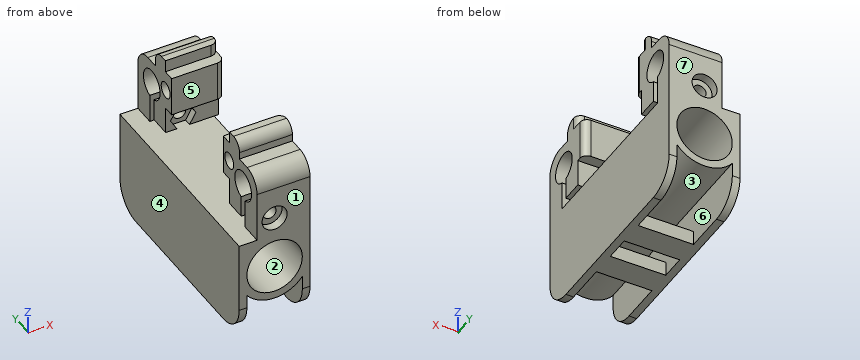
```python
from build123d import *

# Parameters (mm, degrees)
SKETCH_1_W                = 15.5
SKETCH_1_H                = 11.302783866
EXTRUDE_1_DEPTH           = 60
SKETCH_2_R                = 4.2
CUT_EXTRUDE_1_DEPTH       = 90
CUT_EXTRUDE_2_DEPTH       = 40
SKETCH_4_W                = 15.5
SKETCH_4_H                = 19.5
SKETCH_4_H_2              = 7
CUT_EXTRUDE_3_DEPTH       = 6
FILLET_1_R                = 5
FILLET_2_R                = 8
SKETCH_13_R               = 1.8
CUT_EXTRUDE_9_DEPTH       = 75
CUT_EXTRUDE_10_DEPTH      = 34
CUT_EXTRUDE_10_DEPTH_BACK = 2
SKETCH_15_R               = 3.5
CUT_EXTRUDE_11_DEPTH      = 2.5
CUT_EXTRUDE_START         = -2.5
SKETCH_16_R               = 3.5
CUT_EXTRUDE_12_DEPTH      = 2.5
EXTRUDE_2_DEPTH           = 19.8
FILLET_3_R                = 3
SKETCH_18_R               = 2.25
CUT_EXTRUDE_13_DEPTH      = 9
FILLET_4_R                = 2
SKETCH_19_W               = 40.971402115
SKETCH_19_H               = 78.896815639
CUT_EXTRUDE_14_DEPTH      = 5


with BuildPart() as part:
    # Эскиз1 → Бобышка-Вытянуть1 (new body)
    with BuildSketch(Plane(origin=(0, 0, 0), x_dir=(1, 0, 0), z_dir=(0, 1, 0))):
        with BuildLine():
            Line((7.75, 0), (7.75, 6.160154219))
            ThreePointArc((7.75, 6.160154219), (0, 9.9), (-7.75, 6.160154219))
            Line((-7.75, 6.160154219), (-7.75, 1e-08))
            ThreePointArc((-7.75, 1e-08), (5e-09, 7.75), (7.75, 0))
        make_face()
        with BuildLine():
            ThreePointArc((0, -9.9), (4.302584876, -8.916151826), (7.75, -6.160154219))
            Line((7.75, -6.160154219), (7.75, 0))
            ThreePointArc((7.75, 0), (-5e-09, -7.75), (-7.75, 1e-08))
            Line((-7.75, 1e-08), (-7.75, -6.160154219))
            ThreePointArc((-7.75, -6.160154219), (-4.302584876, -8.916151826), (0, -9.9))
        make_face()
        with BuildLine():
            ThreePointArc((7.75, 6.160154219), (9.347058361, 3.262284476), (9.9, 0))
            Line((9.9, 0), (9.9, 18))
            Line((9.9, 18), (-9.9, 18))
            Line((-9.9, 18), (-9.9, 0))
            ThreePointArc((-9.9, 0), (-9.347058361, 3.262284476), (-7.75, 6.160154219))
            Line((-7.75, 6.160154219), (-7.75, 14))
            Line((-7.75, 14), (7.75, 14))
            Line((7.75, 14), (7.75, 6.160154219))
        make_face()
        with BuildLine():
            ThreePointArc((7.75, -6.160154219), (9.347058361, -3.262284476), (9.9, 0))
            ThreePointArc((9.9, 0), (9.347058361, 3.262284476), (7.75, 6.160154219))
            Line((7.75, 6.160154219), (7.75, 0))
            Line((7.75, 0), (7.75, -6.160154219))
        make_face()
        with BuildLine():
            Line((-7.75, 1e-08), (-7.75, 6.160154219))
            ThreePointArc((-7.75, 6.160154219), (-9.347058361, 3.262284476), (-9.9, 0))
            ThreePointArc((-9.9, 0), (-9.347058361, -3.262284476), (-7.75, -6.160154219))
            Line((-7.75, -6.160154219), (-7.75, 1e-08))
        make_face()
        with BuildLine():
            Line((9.9, -29), (9.9, 0))
            ThreePointArc((9.9, 0), (9.347058361, -3.262284476), (7.75, -6.160154219))
            Line((7.75, -6.160154219), (7.75, -9.9))
            Line((7.75, -9.9), (7.75, -11.85))
            Line((7.75, -11.85), (7.75, -23.152783866))
            Line((7.75, -23.152783866), (-7.75, -23.152783866))
            Line((-7.75, -23.152783866), (-7.75, -11.85))
            Line((-7.75, -11.85), (-7.75, -9.9))
            Line((-7.75, -9.9), (-7.75, -6.160154219))
            ThreePointArc((-7.75, -6.160154219), (-9.347058361, -3.262284476), (-9.9, 0))
            Line((-9.9, 0), (-9.9, -29))
            Line((-9.9, -29), (9.9, -29))
        make_face()
        with Locations((0, -17.501391933)):
            Rectangle(SKETCH_1_W, SKETCH_1_H)
        Polygon((7.75, -11.85), (7.75, -9.9), (0, -9.9), (-7.75, -9.9), (-7.75, -11.85), align=None)
        with BuildLine():
            Line((7.75, -9.9), (7.75, -6.160154219))
            ThreePointArc((7.75, -6.160154219), (4.302584876, -8.916151826), (0, -9.9))
            Line((0, -9.9), (7.75, -9.9))
        make_face()
        with BuildLine():
            Line((-7.75, -9.9), (0, -9.9))
            ThreePointArc((0, -9.9), (-4.302584876, -8.916151826), (-7.75, -6.160154219))
            Line((-7.75, -6.160154219), (-7.75, -9.9))
        make_face()
    extrude(amount=EXTRUDE_1_DEPTH)

    # Эскиз2 → Вырез-Вытянуть1 (cut)
    with BuildSketch(Plane(origin=(9.9, 0, 0), x_dir=(0, 0, -1), z_dir=(1, 0, 0))):
        with Locations((-22, 53)):
            Circle(SKETCH_2_R)
        with Locations((-22, 7)):
            Circle(SKETCH_2_R)
    extrude(amount=-CUT_EXTRUDE_1_DEPTH, mode=Mode.SUBTRACT)

    # Эскиз3 → Вырез-Вытянуть2 (cut)
    with BuildSketch(Plane(origin=(9.9, 0, 0), x_dir=(0, 0, -1), z_dir=(1, 0, 0))):
        Polygon((-29, 46), (-29, 14), (-11.85, 14), (-11.85, 8), (-22, 8), (-22, 6), (-9.85, 6), (-9.85, 54), (-22, 54), (-22, 52), (-11.85, 52), (-11.85, 46), align=None)
    extrude(amount=-CUT_EXTRUDE_2_DEPTH, mode=Mode.SUBTRACT)

    # Эскиз4 → Вырез-Вытянуть3 (cut)
    with BuildSketch(Plane(origin=(0, 0, -18), x_dir=(-1, 0, 0), z_dir=(0, 0, -1))):
        with Locations((0, 50.25)):
            Rectangle(SKETCH_4_W, SKETCH_4_H)
        with Locations((0, 30)):
            Rectangle(SKETCH_4_W, SKETCH_4_H_2)
        with Locations((0, 9.75)):
            Rectangle(SKETCH_4_W, SKETCH_4_H)
    extrude(amount=-CUT_EXTRUDE_3_DEPTH, mode=Mode.SUBTRACT)

    # Скругление1
    fillet_1_edges = [part.edges().sort_by_distance(p)[0] for p in [
        (0, 60, 29),
        (0, 0, 29),
    ]]
    fillet(fillet_1_edges, radius=FILLET_1_R)

    # Скругление2
    fillet_2_edges = [part.edges().sort_by_distance(p)[0] for p in [
        (-8.825, 60, -18),
        (-8.825, 0, -18),
        (8.825, 0, -18),
        (8.825, 60, -18),
    ]]
    fillet(fillet_2_edges, radius=FILLET_2_R)

    # Эскиз13 → Вырез-Вытянуть9 (cut)
    with BuildSketch(Plane.XZ):
        with Locations(Location((0, 14.920784389, 0), (0, 0, 270))):
            Circle(SKETCH_13_R)
    extrude(amount=-CUT_EXTRUDE_9_DEPTH, mode=Mode.SUBTRACT)

    # Эскиз14 → Вырез-Вытянуть10 (cut, two sides: drawn at the far end of the back side and taken through both)
    with BuildSketch(Plane(origin=(0, 14, 0), x_dir=(1, 0, 0), z_dir=(0, 1, 0)).offset(-CUT_EXTRUDE_10_DEPTH_BACK)):
        Polygon((-1.772918194, -17.991568778), (1.772918194, -17.991568778), (3.545836387, -14.920784389), (1.772918194, -11.85), (-1.772918194, -11.85), (-3.545836387, -14.920784389), align=None)
    extrude(amount=CUT_EXTRUDE_10_DEPTH + CUT_EXTRUDE_10_DEPTH_BACK, mode=Mode.SUBTRACT)

    # Эскиз15 → Вырез-Вытянуть11 (cut)
    with BuildSketch(Plane(origin=(0, 60, 0), x_dir=(1, 0, 0), z_dir=(0, 1, 0))):
        with Locations(Location((0, -14.920784389, 0), (0, 0, 270))):
            Circle(SKETCH_15_R)
    extrude(amount=-CUT_EXTRUDE_11_DEPTH, mode=Mode.SUBTRACT)

    # Эскиз16 → Вырез-Вытянуть12 (cut)
    with BuildSketch(Plane.XZ.offset(CUT_EXTRUDE_START)):
        with Locations(Location((0, 14.920784389, 0), (0, 0, 90))):
            Circle(SKETCH_16_R)
    extrude(amount=CUT_EXTRUDE_12_DEPTH, mode=Mode.SUBTRACT)

    # Эскиз17 → Бобышка-Вытянуть2 (add)
    with BuildSketch(Plane(origin=(9.9, 0, 0), x_dir=(0, 0, -1), z_dir=(1, 0, 0))):
        Polygon((-30.6, 43), (-19.4, 43), (-19.4, 46), (-29, 46), (-29, 51.15), (-34, 51.15), (-34, 46.15), (-30.6, 46.15), align=None)
        Polygon((-29, 14), (-19.4, 14), (-19.4, 17), (-28.462723747, 17), (-30.6, 17), (-30.6, 13.85), (-34, 13.85), (-34, 8.85), (-29.808389015, 8.85), (-29, 8.85), align=None)
    extrude(amount=-EXTRUDE_2_DEPTH)

    # Скругление3
    fillet_3_edges = [part.edges().sort_by_distance(p)[0] for p in [
        (0, 51.15, 34),
        (0, 8.85, 34),
    ]]
    fillet(fillet_3_edges, radius=FILLET_3_R)

    # Эскиз18 → Вырез-Вытянуть13 (cut)
    with BuildSketch(Plane.ZY.offset(9.9)):
        with Locations((25, 14)):
            Circle(SKETCH_18_R)
        with Locations((25, 46)):
            Circle(SKETCH_18_R)
    extrude(amount=-CUT_EXTRUDE_13_DEPTH, mode=Mode.SUBTRACT)

    # Скругление4
    fillet_4_edges = [part.edges().sort_by_distance(p)[0] for p in [
        (9.9, 13.85, 32.3),
        (9.9, 17, 25),
        (9.9, 43, 25),
        (9.9, 46.15, 32.3),
    ]]
    fillet(fillet_4_edges, radius=FILLET_4_R)

    # Эскиз19 → Вырез-Вытянуть14 (cut)
    with BuildSketch(Plane.ZY.offset(9.9)):
        with Locations((30.335701058, 24.667257597)):
            Rectangle(SKETCH_19_W, SKETCH_19_H)
    extrude(amount=-CUT_EXTRUDE_14_DEPTH, mode=Mode.SUBTRACT)


solid = part.part
```
Model file for the job. Use its own axes, mm. Face numbers are marked on the shaded views. A direction names the side the tool comes from. Coordinates: 2 decimals unless noted, no trailing zeros. Write each loop counter-clockwise with the first axis right and the second up, starting at its lowest first coordinate (ties: lowest second). Pieces come first, ordered by that corner, then holes. Notation, with made-up numbers: (74.5, 9) - (89.5, 9) arc R22 ccw to (89.5, 34) - close; hole circle Ø3 at (59.25, -24.5). An arc over 180 degrees is marked (long way). One line per item, written item: value. Start each with the question number.
1. Slice it at C-C (z = -4). Write the cut outline in (x, y), plus the area to 3 significant figures.
2. Flat gauge pins, fed straight in: pin 1 (1.9 mm diameter, centred on x = 2.5, y = 52.5, fed in from +Z); pin 2 (2 mm diameter, centred on x = 0.5, y = 37.5, fed in from +Z); pin 3 (2 mm diameter, centred on y = 45, z = 24.5, fed in from -X). Where does each tip first touch, or does it go through?
3. Slice it at B-B (y = 53). Write the cut outline in (x, z).
4. Tool access for the marked faces 5, 6 and 7: list every direction of +Z, -Z, +X, -X, +Y, -Y with a clear straight run to the whole face (end or side of a thin tool).
5. Mould opens along X. For the marked faces 1, 2, 3 and 4 say: released by +X, released by -X, zero draft, split by the parting line, or undercut.
6. Probe line 1 (Z direction, x = 0, y = 21); line 2 (Y direction, x = 3.5, z = 23.5); line 3 (Y direction, x = -1.5, z = 12.5). List the from-to ranges inside material, lowest first. Write a range as from..to.
7. Slice it at D-D (y = 36). Write the cut outline in (x, z).
8. Slice it at A-A (z = 22). Write the cut outline in (x, y), plus the area to 3 significant figures.
Answers below:
1. outline: (-9.9, 0) - (-6.64, 0) - (-6.64, 60) - (-9.9, 60) - close; (6.64, 0) - (9.9, 0) - (9.9, 60) - (6.64, 60) - close
1. area: 391 mm^2
2. pin 1: stops at z = 29
2. pin 2: stops at z = 9.85
2. pin 3: stops at x = -0.9
3. outline: (-9.9, -17.94) - (-7.75, -17.94) - (-7.75, -6.16) arc R9.9 ccw to (7.75, -6.16) - (7.75, -17.94) - (9.9, -17.94) - (9.9, 9.85) - (-9.9, 9.85) - close; (-4.9, 26.2) - (9.9, 26.2) - (9.9, 29) - (-4.9, 29) - close; hole circle Ø15.5 at (0, 0)
4. face 5: +Z, +X, -X
4. face 6: none
4. face 7: +Z, -Z, +X, -X, +Y
5. face 1: zero draft
5. face 2: undercut
5. face 3: undercut
5. face 4: released by -X
6. line 1: z = -18..-14, -9.9..-7.75, 7.75..9.85
6. line 2: y = 0..3.08, 10.92..17, 43..49.08, 56.92..60
6. line 3: y = 2.5..6, 8..12, 48..52, 54..57.5
7. outline: (-9.9, -18) - (9.9, -18) - (9.9, 9.85) - (-9.9, 9.85) - close; hole (-7.75, -14) - (7.75, -14) - (7.75, -6.16) arc R9.9 cw to (-7.75, -6.16) - close; hole circle Ø15.5 at (0, 0)
8. outline: (-4.9, 0) - (9.9, 0) - (9.9, 2.8) - (-4.9, 2.8) - close; (-4.9, 11.2) - (9.9, 11.2) - (9.9, 15) arc R2 ccw to (7.9, 17) - (-4.9, 17) - close; (-4.9, 43) - (7.9, 43) arc R2 ccw to (9.9, 45) - (9.9, 48.8) - (-4.9, 48.8) - close; (-4.9, 57.2) - (9.9, 57.2) - (9.9, 60) - (-4.9, 60) - close
8. area: 253 mm^2
